Work out the finished part from the listing and answer in its coordinate system (mm). A direction names the side the tool comes from. Give positions to 0.01 mm unless a question says otherwise; leave off trailing zeros. Order: outer loops, then holes, each group sorted by start corner. A loop starts at its lowest first (then second) coordinate and runs counter-clockwise, first axis right, second up. Notation, with made-up numbers: (45.5, 53) -> (97.5, 53) arc R30 ccw to (97.5, 77) -> close; hole circle Ø10 at (59, 14.5). An arc over 180 degrees is marked (long way). Use a Markdown table: item, result. Add a question column.
```python
from build123d import *

# Parameters (mm, degrees)
F0_R     = 28.5
F1_DEPTH = 3
F2_R     = 26.1
F2_R_2   = 23.9
F3_DEPTH = 1


with BuildPart() as f1:
    # F0 (on Top) → F1 (new body)
    with BuildSketch(Plane.XY):
        Circle(F0_R)
    extrude(amount=F1_DEPTH)

    # F2 (on face) → F3 (cut)
    with BuildSketch(Plane.XY.offset(3)):
        Circle(F2_R)
        Circle(F2_R_2, mode=Mode.SUBTRACT)
    extrude(amount=-F3_DEPTH, mode=Mode.SUBTRACT)


solid = f1.part
```
1) The part is cut by section A-A, the plane y = 0. Determine the outline of the cut face in (x, z), then the cut area to 3 significant figures.
2) Which of the six approach directions +Z, -Z, +X, -X, +Y, -Y give full straight-line access (tool end or side, diameter ignored) to faces 5 (the cylindrical face through (12.85, 20.15, 2.51)), 6 (the flat face through (0, 0, 0))?
3) The part is cut by section D-D, the plane x = -25. Determine the outline of the cut face in (y, z).
4) Determine the mould class of faces 1 (the cylindrical face through (26.327, -10.916, 1.479)), 2 (the flat face through (11.48, -21.14, 2)), 3 (the cylindrical face through (-19.237, 17.64, 2.507)), 4 (the flat face through (13, -23, 3)) for opening direction Y: released by +Y, released by -Y, zero draft, split by the parting line, or undercut.
5) Flat-ended cylindrical pins translate along their axes: pin 1 (1 mm diameter, centred on y = -6, z = 2, fed in from -X); pin 2 (1.5 mm diameter, centred on y = -22.5, z = 2, fed in from +X). Find the tip coordinate at first contact, or state that the pin passes through.
6) The part is cut by section C-C, the plane z = 0.95. Determine the outline of the cut face in (x, y), then the cut area to 3 significant figures.
7) Straight lines are drawn through the part: line 1 (X direction, y = 7, z = 2.25); line 2 (X direction, y = -4, z = 2.5); line 3 (Y direction, x = -10.5, z = 2.4). For each, find the intervals that lie inside material, in ascending order.
A:
| question | item | result |
|---|---|---|
| 1 | outline | (-28.5, 0) -> (28.5, 0) -> (28.5, 3) -> (26.1, 3) -> (26.1, 2) -> (23.9, 2) -> (23.9, 3) -> (-23.9, 3) -> (-23.9, 2) -> (-26.1, 2) -> (-26.1, 3) -> (-28.5, 3) -> close |
| 1 | area | 167 mm^2 |
| 2 | face 5 | +Z |
| 2 | face 6 | -Z, +X, -X, +Y, -Y |
| 3 | outline | (-13.68, 0) -> (13.68, 0) -> (13.68, 3) -> (7.5, 3) -> (7.5, 2) -> (-7.5, 2) -> (-7.5, 3) -> (-13.68, 3) -> close |
| 4 | face 1 | split by the parting line |
| 4 | face 2 | undercut |
| 4 | face 3 | undercut |
| 4 | face 4 | zero draft |
| 5 | pin 1 | x = -27.96 |
| 5 | pin 2 | x = 18.42 |
| 6 | outline | circle Ø57 at (0, 0) |
| 6 | area | 2,550 mm^2 |
| 7 | line 1 | -27.63 to -25.14, -22.85 to 22.85, 25.14 to 27.63 |
| 7 | line 2 | -28.22 to -25.79, -23.56 to 23.56, 25.79 to 28.22 |
| 7 | line 3 | -26.5 to -23.89, -21.47 to 21.47, 23.89 to 26.5 |
